For this review, take the finished solid that the model builds, in its own axes (mm). Coordinates: 2 decimals unless noted, no trailing zeros. Order: outer loops, then holes, each group sorted by start corner. A loop starts at its lowest first (then second) coordinate and runs counter-clockwise, first axis right, second up.
from build123d import *

# Parameters (mm, degrees)
BOSS_EXTRUDE1_DEPTH = 1.5


with BuildPart() as part:
    # Sketch1 → Boss-Extrude1 (new body, symmetric)
    with BuildSketch(Plane.XY):
        Polygon((65, -147.5), (75, -147.5), (75, -160), (75, -190), (62.5, -190), (62.5, -160), (15, -160), (-15, -160), (-15, 160), (15, 160), (15, -147.5), align=None)
    extrude(amount=BOSS_EXTRUDE1_DEPTH, both=True)


solid = part.part
1. To check wall thickness, follow L1, parallel to X at y = -166.5, z = -0.55; L2, parallel to X at y = 97, z = -0.4; L3, parallel to Y at x = 41, z = -0.5. State the ranges of each line that lie inside material, in increasing order.
Answer below:
L1: x = 62.5 to 75
L2: x = -15 to 15
L3: y = -160 to -147.5
2. Take a section at B-B, the plane x = 33.5. Give the boundary of the cut face in (y, z), plus the area to 3 significant figures.
Answer below:
outline: (-160, -1.5) - (-147.5, -1.5) - (-147.5, 1.5) - (-160, 1.5) - close
area: 37.5 mm2
3. Take a section at A-A, the plane z = -0.75. Give the boundary of the cut face in (x, y), plus the area to 3 significant figures.
Answer below:
outline: (-15, -160) - (62.5, -160) - (62.5, -190) - (75, -190) - (75, -147.5) - (15, -147.5) - (15, 160) - (-15, 160) - close
area: 10,700 mm2
4. Clearance check with a flat-ended pin moving along its axis: pin 1 Ø1.5 at (x, z) = (23.5, 0.5) entering from -Y. State where the tip first meets the part, or that it passes through.
Answer below:
pin 1: stops at y = -160
5. Take a section at C-C, the plane y = 106.5. Give the boundary of the cut face in (x, z), plus the area to 3 significant figures.
Answer below:
outline: (-15, -1.5) - (15, -1.5) - (15, 1.5) - (-15, 1.5) - close
area: 90.0 mm2
